from build123d import *

# Parameters (mm, degrees)
F0_W     = 70
F0_H     = 12
F1_DEPTH = 5
F2_R     = 4.025
F3_DEPTH = 25.4
F5_DEPTH = 69.977
F6_R     = 4.025
F7_DEPTH = 25.4
F9_DEPTH = 25.4


with BuildPart() as f1:
    # F0 (on Front) → F1 (new body)
    with BuildSketch(Plane.XZ):
        Rectangle(F0_W, F0_H)
    extrude(amount=F1_DEPTH)

    # F2 (on face) → F3 (cut)
    with BuildSketch(Plane.XZ.offset(5)):
        with Locations((-26.5, 0)):
            Circle(F2_R)
        with Locations((26.5, 0)):
            Circle(F2_R)
    extrude(amount=-F3_DEPTH, mode=Mode.SUBTRACT)

    # F4 (on face) → F5 (join)
    with BuildSketch(Plane.YZ.offset(35)):
        with BuildLine():
            Line((-80.10874, -86.10874), (0, -6))
            Line((0, -6), (-5, -6))
            Line((-5, -6), (-5, -2.019744))
            Line((-5, -2.019744), (-84.598868, -81.618612))
            ThreePointArc((-84.598868, -81.618612), (-83.067369, -84.577241), (-80.10874, -86.10874))
        make_face()
    extrude(amount=-F5_DEPTH)

    # F6 (on face) → F7 (cut)
    with BuildSketch(Plane(origin=(0, 0, 0), x_dir=(-1, 0, 0), z_dir=(0, 1, 0))):
        with Locations((26.5, 0)):
            Circle(F6_R)
        with Locations((-26.5, 0)):
            Circle(F6_R)
    extrude(amount=-F7_DEPTH, mode=Mode.SUBTRACT)

    # F8 (on face) → F9 (cut)
    with BuildSketch(Plane(origin=(0, 3, -3), x_dir=(-1, 0, 0), z_dir=(0, 0.707107, -0.707107))):
        Polygon((-3.665127, -67.304638), (-28.65, -23.425769), (-28.65, -111.183507), align=None)
        Polygon((-0.0115, -60.888074), (28.627, -10.592641), (-28.65, -10.592641), align=None)
        Polygon((28.627, -111.183507), (28.627, -23.425769), (3.642127, -67.304638), align=None)
        Polygon((-21.342745, -111.183507), (21.319745, -111.183507), (-0.0115, -73.721202), align=None)
    extrude(amount=-F9_DEPTH, mode=Mode.SUBTRACT)


solid = f1.part
The model under review builds one solid part; all positions refer to its coordinate system, in mm. Round coordinates to 2 decimals unless told otherwise and drop trailing zeros. Order: outer loops, then holes, each group sorted by start corner. A loop starts at its lowest first (then second) coordinate and runs counter-clockwise, first axis right, second up. Notation, with made-up numbers: (32.5, 56.5) -> (37.5, 56.5) arc R8 ccw to (37.5, 65.5) -> close; hole circle Ø1 at (37, 58.5). An arc over 180 degrees is marked (long way). Use CSV: the item, a comma, the result in double quotes. Start each with the question number.
(1) Consider section C-C on z = -61. Write out the cut boundary in (x, y).
(2) Consider section D-D on x = -9. Write out the cut boundary in (y, z), and give its area (3 significant figures).
(3) Mouldability with a two-part tool opening along X and no side actions: class faces 1 (the face through (0.501, -83.101, -84.544)), 2 (the face through (-16.31, -31.07, -32.65)), 3 (the face through (-34.977, -42, -44)) as pulls with the +X half, pulls with the -X half, needs draft (parallel to the pull), parting line crosses it, or undercut.
(4) Consider section B-B on y = -21. Write out the cut boundary in (x, z).
(5) Wall thickness on probe 1 along X at (y, z) = (-1.5, 0) (3 decimals); probe 2 along X at (y, z) = (-50, -50.5); probe 3 along Z at (x, y) = (26.5, -3) (3 decimals): over which ranges is each line inside the solid? List them lowest first. Write a range as from..to.
(6) Insertion check: pin 1 (9.5 mm diameter, centred on x = 5, z = 0.5, fed in from -Y); pin 2 (1.5 mm diameter, centred on x = 26.5, z = -16, fed in from -Y); pin 3 (4 mm diameter, centred on x = 20.5, y = -18.5, fed in from +Z). Each pin has a flat end and moves straight along its axis. Give the tip position at first contact, or say it passes through.
(7) Consider section A-A on z = 0. Write out the cut boundary in (x, y) (3 decimals).
Responses:
1,outline,"(-34.98, -63.98) -> (-28.63, -63.98) -> (-28.63, -55) -> (-34.98, -55) -> close; (-15.64, -63.98) -> (-8.33, -63.98) -> (-4.72, -55) -> (-12.02, -55) -> close; (4.74, -55) -> (8.36, -63.98) -> (15.66, -63.98) -> (12.05, -55) -> close; (28.65, -63.98) -> (35, -63.98) -> (35, -55) -> (28.65, -55) -> close"
2,outline,"(-84.6, -81.62) arc R5.5 ccw to (-80.11, -86.11) -> (-75.62, -81.62) -> (-80.11, -77.13) -> close; (-64.81, -61.83) -> (-60.32, -66.32) -> (-51.25, -57.25) -> (-55.74, -52.76) -> close; (-42.43, -39.45) -> (-37.94, -43.94) -> (-28.86, -34.86) -> (-33.35, -30.37) -> close; (-8.98, -6) -> (-4.49, -10.49) -> (0, -6) -> (0, 6) -> (-5, 6) -> (-5, -2.02) -> close"
2,area,"296 mm²"
3,face 1,"needs draft"
3,face 2,"undercut"
3,face 3,"pulls with the -X half"
4,outline,"(-34.98, -27) -> (-28.63, -27) -> (-28.63, -18.02) -> (-34.98, -18.02) -> close; (-26.26, -18.02) -> (-22.64, -27) -> (-15.33, -27) -> (-18.95, -18.02) -> close; (15.36, -27) -> (22.66, -27) -> (26.28, -18.02) -> (18.97, -18.02) -> close; (28.65, -27) -> (35, -27) -> (35, -18.02) -> (28.65, -18.02) -> close"
5,probe 1,"-35..-30.525, -22.475..22.475, 30.525..35"
5,probe 2,"-34.98..-28.63, -5.78..5.81, 28.65..35"
5,probe 3,"-9..-4.025, 4.025..6"
6,pin 1,"y = -7.23"
6,pin 2,"y = -19.73"
6,pin 3,"z = -14.23"
7,outline,"(-35, -5) -> (-30.525, -5) -> (-30.525, 0) -> (-35, 0) -> close; (-22.475, -5) -> (22.475, -5) -> (22.475, 0) -> (-22.475, 0) -> close; (30.525, -5) -> (35, -5) -> (35, 0) -> (30.525, 0) -> close"
